The listing builds one solid part. Answer for the finished solid, in the listing's coordinates (mm). Face numbers are marked on the shaded views. Give positions to 0.01 mm unless a question says otherwise; leave off trailing zeros. Write each loop counter-clockwise with the first axis right and the second up, starting at its lowest first coordinate (ties: lowest second). Pieces come first, ordered by that corner, then holes. Notation, with made-up numbers: (54.5, -38.75) -> (106.5, -38.75) arc R25 ccw to (106.5, -14.75) -> close; hole circle Ø2 at (-21, -34.75). An arc over 180 degrees is marked (long way). One line per question, with ' | ' between items.
from build123d import *

# Parameters (mm, degrees)
F0_W           = 44.45
F0_H           = 11.43
F1_DEPTH       = 6.35
F2_D           = 3.937
F2_DEPTH       = 6.35
F2_CBORE_D     = 7.256526
F2_CBORE_DEPTH = 1.5875
F3_SIZE        = 1.5


with BuildPart() as f1:
    # F0 (on Front) → F1 (new body)
    with BuildSketch(Plane.XZ):
        Rectangle(F0_W, F0_H)
    extrude(amount=F1_DEPTH)

    # F2
    with Locations(Plane(origin=(0, 0, 0), x_dir=(1, 0, 0), z_dir=(0, 1, 0))):
        with Locations((-11.43, 0), (11.43, 0)):
            CounterBoreHole(F2_D / 2, F2_CBORE_D / 2, F2_CBORE_DEPTH, depth=F2_DEPTH)

    # F3
    f3_edges = [f1.edges().sort_by_distance(p)[0] for p in [
        (0, 0, 5.715),
        (0, 0, -5.715),
        (22.225, 0, 0),
        (-22.225, 0, 0),
        (22.225, -3.175, -5.715),
        (22.225, -3.175, 5.715),
        (-22.225, -3.175, 5.715),
        (-22.225, -3.175, -5.715),
    ]]
    chamfer(f3_edges, length=F3_SIZE)


solid = f1.part
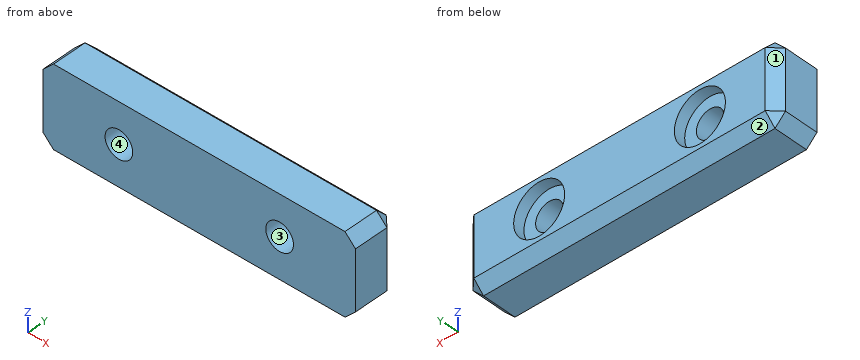
Item 1: Determine the mould class of the marked faces 1, 2, 3 and 4 for opening direction Z: pulls with the +Z half, pulls with the -Z half, needs draft (parallel to the pull), parting line crosses it, or undercut.
Answers below:
face 1: needs draft | face 2: pulls with the -Z half | face 3: undercut | face 4: undercut
Item 2: Find section D-D (x = 1.5). Write down the section's boundary in (y, z) (3 decimals).
Answers below:
outline: (-6.35, -5.715) -> (-1.5, -5.715) -> (0, -4.215) -> (0, 4.215) -> (-1.5, 5.715) -> (-6.35, 5.715) -> close
Item 3: Flat-ended cylindrical pins translate along their axes: pin 1 (5 mm diameter, centred on x = -11.43, z = 0, fed in from -Y); pin 2 (3 mm diameter, centred on x = 11.43, z = 0, fed in from +Y); pin 3 (3 mm diameter, centred on x = 10, z = 0.5, fed in from +Y). Find the tip coordinate at first contact, or state that the pin passes through.
Answers below:
pin 1: y = -6.35 | pin 2: through | pin 3: y = -1.59
Item 4: Consider line 1 (X direction, y = -3, z = -1) (3 decimals); line 2 (Z direction, x = 11.43, y = -4.15) (1 decimal); line 3 (X direction, y = -1, z = -2) (3 decimals). Determine where each line is inside the solid, lowest interval first. Write a range as [from, to].
Answers below:
line 1: [-22.225, -13.126], [-9.734, 9.734], [13.126, 22.225] | line 2: [-5.7, -2], [2, 5.7] | line 3: [-21.725, -14.457], [-8.403, 8.403], [14.457, 21.725]
Item 5: Find section C-C (y = -5.25). Write down the section's boundary in (x, z) (1 decimal).
Answers below:
outline: (-22.2, -4.2) -> (-20.7, -5.7) -> (20.7, -5.7) -> (22.2, -4.2) -> (22.2, 4.2) -> (20.7, 5.7) -> (-20.7, 5.7) -> (-22.2, 4.2) -> close; hole circle Ø3.9 at (-11.4, 0); hole circle Ø3.9 at (11.4, 0)
Item 6: Find section A-A (z = 0). Count the separate pieces of the cut face and the enclosed holes in it, then the cut area to 3 significant figures.
Answers below:
separate pieces: 3 | enclosed holes: 0 | area: 219 mm²
